Design review of the part built by this model. Coordinates are the model's own, in mm. A direction names the side the tool comes from. Give positions to 0.01 mm unless a question says otherwise; leave off trailing zeros. Write each loop counter-clockwise with the first axis right and the second up, starting at its lowest first coordinate (ties: lowest second). Pieces come first, ordered by that corner, then holes. Notation, with made-up numbers: (88.25, -38) - (120.25, -38) arc R27 cw to (120.25, 1) - close; hole circle Ø10 at (-37, -25). An arc over 180 degrees is marked (long way). Use a Markdown table: item, result. Add a question column.
```python
from build123d import *

# Parameters (mm, degrees)
F0_W      = 191.0914182663
F0_H      = 192.8930431604
F1_DEPTH  = 25.4
F2_W      = 25.4
F2_H      = 25.5114277713
F3_DEPTH  = 25.4
F4_W      = 125.7558986545
F4_H      = 7.1474313736
F4_H_2    = 192.8930431604
F4_W_2    = 50.9491413832
F5_DEPTH  = 25.4
F7_DEPTH  = 25.4
F9_W      = 164.3103808165
F9_H      = 10.6280595064
F10_DEPTH = 25.4


with BuildPart() as f1:
    # F0 (on Front) → F1 (new body)
    with BuildSketch(Plane.XZ):
        with Locations((-0.6164610386, -0.6837919354)):
            Rectangle(F0_W, F0_H)
        Polygon((0, 75.5859687924), (74.6201202273, 75.5859687924), (74.6201202273, 11.123508215), (81.607028842, -13.4125072509), (74.6201202273, -13.2084926445), (74.6201202273, -76.0672464967), (0, -76.0672464967), (-77.7053460479, -76.0672464967), (-77.7053460479, -8.7606571615), (-77.7053460479, 12.5154424459), (-77.7053460479, 75.5859687924), align=None, mode=Mode.SUBTRACT)
    extrude(amount=F1_DEPTH)

    # F2 (on face) → F3 (join)
    with BuildSketch(Plane(origin=(71.9530620256, 0, 20.4894502783), x_dir=(0, -1, 0), z_dir=(-0.9617656717, 0, -0.2738736803))):
        with Locations((12.7, -22.4939924905)):
            Rectangle(F2_W, F2_H)
    extrude(amount=F3_DEPTH)

    # F4 (on face) → F5 (join)
    with BuildSketch(Plane.XZ.offset(25.4)):
        with Locations((32.0512987673, -100.7040292025)):
            Rectangle(F4_W, F4_H)
        with Locations((32.0512987673, -0.6837919354)):
            Rectangle(F4_W, F4_H_2)
        Polygon((-30.8266505599, -104.2777448893), (-30.8266505599, -97.1303135157), (-81.7757919431, -97.1303135157), (-81.7757919431, 95.7627296448), (-113.723911345, 95.7627296448), (-113.723911345, -104.2777448893), align=None)
        with Locations((-56.3012212515, -0.6837919354)):
            Rectangle(F4_W_2, F4_H_2)
    extrude(amount=F5_DEPTH)

    # F6 (on face) → F7 (join)
    with BuildSketch(Plane(origin=(0, -25.4, 0), x_dir=(-1, 0, 0), z_dir=(0, 1, 0))):
        Polygon((-98.9333018661, 95.3389704227), (-94.9292480946, -97.1303135157), (113.723911345, -97.1303135157), (113.723911345, 86.9726911187), align=None)
    extrude(amount=F7_DEPTH)

    # F9 (on face) → F10 (join)
    with BuildSketch(Plane(origin=(0, 0, 0), x_dir=(-1, 0, 0), z_dir=(0, 1, 0))):
        Polygon((-95.9361866117, 86.4189863205), (-95.9361866117, -96.4786112309), (73.3251571655, -96.4786112309), (73.3251571655, 86.4189863205), (68.3741942048, 86.4189863205), align=None)
        with Locations((-13.7809962034, 91.7330160737)):
            Rectangle(F9_W, F9_H)
    extrude(amount=F10_DEPTH)


solid = f1.part
```
(1) For line 1 along Z through (x, y) = (12.5, -8); line 2 along X through (y, z) = (13, -49.5); line 3 along Y through (x, z) = (-96, -88), list the stretches that pass through material, from the lowest coordinate up.
(2) Add section B-B (z = -39). State the section outline as (x, y) points, and give its area (3 significant figures).
(3) Add section C-C (y = -14.5). State the section outline as (x, z) points, and give its area (3 significant figures).
(4) Tool access review of faces 1 (the face through (95.936, 13, 2)), 2 (the face through (-96.162, -13, 92)), 3 (the face through (-11, -13, -97.13)): name each direction out of +Z, -Z, +X, -X, +Y, -Y from which nothing blocks a thin tool from reaching the whole face with its end or side.
(5) Add section D-D (x = -93). State the section outline as (y, z) points, and give its area (3 significant figures).
(6) Insertion check: pin 1 (12.5 mm diameter, centred on y = 15.5, z = -26, fed in from +X); pin 2 (10 mm diameter, centred on x = 64.5, y = -37, fed in from +Z); pin 3 (2 mm diameter, centred on x = -39.5, z = -101, fed in from +Y). Each pin has a flat end and moves straight along its axis. Give the tip position at first contact, or say it passes through.
(7) Add section A-A (x = -59). State the section outline as (y, z) points.
Answers follow:
| question | item | result |
|---|---|---|
| 1 | line 1 | -97.13 to 95.76 |
| 1 | line 2 | -73.33 to 95.94 |
| 1 | line 3 | -50.8 to 0 |
| 2 | outline | (-113.72, -50.8) - (94.93, -50.8) - (94.93, -25.4) - (96.14, -25.4) - (96.14, 0) - (95.94, 0) - (95.94, 25.4) - (-73.33, 25.4) - (-73.33, 0) - (-113.72, 0) - close |
| 2 | area | 14,900 mm^2 |
| 3 | outline | (-113.72, -97.13) - (94.93, -97.13) - (98.93, 95.34) - (94.93, 95.18) - (94.93, 95.76) - (-96.16, 95.76) - (-96.16, 87.66) - (-113.72, 86.97) - close |
| 3 | area | 40,500 mm^2 |
| 4 | face 1 | +Z, -Z, +X, +Y |
| 4 | face 2 | +Z, -X, +Y |
| 4 | face 3 | -Z, +X, -X, +Y |
| 5 | outline | (-50.8, -104.28) - (-25.4, -104.28) - (-25.4, -97.13) - (0, -97.13) - (0, 95.76) - (-50.8, 95.76) - close |
| 5 | area | 9,980 mm^2 |
| 6 | pin 1 | x = 95.94 |
| 6 | pin 2 | z = 95.76 |
| 6 | pin 3 | y = -25.4 |
| 7 | outline | (-50.8, -104.28) - (-25.4, -104.28) - (-25.4, -97.13) - (0, -97.13) - (0, -96.48) - (25.4, -96.48) - (25.4, 97.05) - (0, 97.05) - (0, 95.76) - (-50.8, 95.76) - close |
